from build123d import *

# Parameters (mm, degrees)
F0_W     = 30
F0_H     = 150
F1_DEPTH = 2


with BuildPart() as f1:
    # F0 (on Top) → F1 (new body)
    with BuildSketch(Plane.XY):
        with Locations((15, 75)):
            Rectangle(F0_W, F0_H)
        Polygon((6, 9), (6, 141), (12, 141), (12, 136.5), (18, 136.5), (18, 141), (24, 141), (24, 9), (18, 9), (18, 13.5), (12, 13.5), (12, 9), align=None, mode=Mode.SUBTRACT)
    extrude(amount=F1_DEPTH)


solid = f1.part
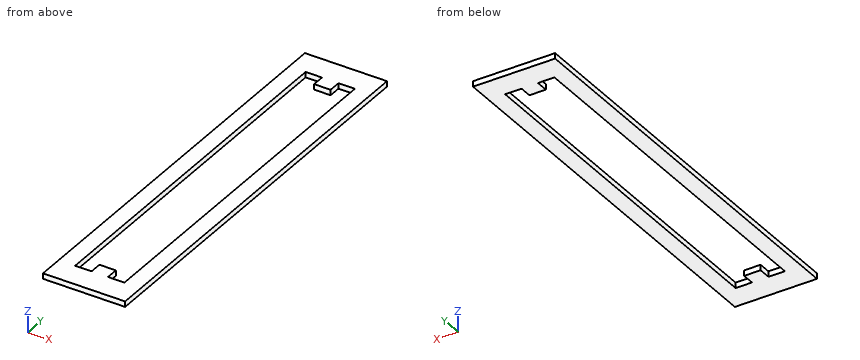
Can you work these out from the model? Positions are in its coordinate system, mm. Give positions to 0.01 mm unless a question says otherwise; leave off trailing zeros. Write each loop counter-clockwise with the first axis right and the second up, starting at its lowest first coordinate (ties: lowest second). Pieces come first, ordered by that corner, then holes. Notation, with made-up numbers: (-38, 60) -> (-22, 60) arc R13 cw to (-22, 74) -> close; hole circle Ø11 at (-29.5, 19). An arc over 180 degrees is marked (long way). Answer as a JSON object with one key per item and string values. Group by question number.
Item 1: Suppose I cut it at C-C (z = 0.75). Please give me the cut outline in (x, y), plus the area to 3 significant figures.
Item 2: I'm going to push flat-ended pins straight in: P1, Ø0.6, axis at x = 22, z = 1.5, coming from the -Y side; P2, Ø1, axis at x = 7.5, y = 92, coming from the +Z side. Where does each tip first touch, or does it pass through?
Item 3: Suppose I cut it at B-B (x = 16). Please give me the cut outline in (y, z), plus the area to 3 significant figures.
Item 4: Please list where these lines run through material, in increasing order: line 1 (Y direction, x = 19.5, z = 1.25); line 2 (Y direction, x = 17.5, z = 0.15); line 3 (X direction, y = 122.5, z = 1.8). Write a range as [from, to].
Item 5: Suppose I cut it at A-A (y = 127). Please give me the cut outline in (x, z), plus the area to 3 significant figures.
Findings:
{
 "1": {"outline": "(0, 0) -> (30, 0) -> (30, 150) -> (0, 150) -> close; hole (6, 9) -> (12, 9) -> (12, 13.5) -> (18, 13.5) -> (18, 9) -> (24, 9) -> (24, 141) -> (18, 141) -> (18, 136.5) -> (12, 136.5) -> (12, 141) -> (6, 141) -> close", "area": "2,180 mm²"},
 "2": {"P1": "stops at y = 0", "P2": "passes through"},
 "3": {"outline": "(0, 0) -> (13.5, 0) -> (13.5, 2) -> (0, 2) -> close; (136.5, 0) -> (150, 0) -> (150, 2) -> (136.5, 2) -> close", "area": "54.0 mm²"},
 "4": {"line 1": "y = [0, 9], [141, 150]", "line 2": "y = [0, 13.5], [136.5, 150]", "line 3": "x = [0, 6], [24, 30]"},
 "5": {"outline": "(0, 0) -> (6, 0) -> (6, 2) -> (0, 2) -> close; (24, 0) -> (30, 0) -> (30, 2) -> (24, 2) -> close", "area": "24.0 mm²"}
}
